Input: part model. Units: mm. Frame: model coordinates. Face numbers are marked on the shaded views. A direction names the side the tool comes from. Round coordinates to 2 decimals unless told otherwise and drop trailing zeros. Write each loop counter-clockwise with the first axis right and the second up, starting at its lowest first coordinate (ties: lowest second). Pieces come first, ordered by that corner, then holes. Notation, with made-up numbers: (11, -22) -> (28, -22) arc R24 cw to (28, 4) -> close; hole circle Ø5 at (65, -19). An arc over 180 degrees is marked (long way). Use CSV: the item, a comma, the result in double quotes.
```python
from build123d import *

# Parameters (mm, degrees)
BOSS_EXTRUDE1_DEPTH = 38.1
SKETCH2_W           = 28.575
SKETCH2_H           = 22.225
CUT_EXTRUDE1_DEPTH  = 39.1
SKETCH3_R           = 1.5875
CUT_EXTRUDE2_DEPTH  = 37.5125
SKETCH4_R           = 1.8415
CUT_EXTRUDE3_DEPTH  = 37.5125
CIRPATTERN1_COUNT   = 8
FILLET1_R           = 2.54
FILLET2_R           = 2.54


with BuildPart() as part:
    # Sketch1 → Boss-Extrude1 (new body)
    with BuildSketch(Plane.XY):
        Polygon((0, 0), (0, 31.75), (33.3375, 31.75), (33.3375, 36.5125), (-4.7625, 36.5125), (-4.7625, 0), align=None)
    extrude(amount=BOSS_EXTRUDE1_DEPTH)

    # Sketch2 → Cut-Extrude1 (cut, through all)
    with BuildSketch(Plane.ZY.offset(4.7625)):
        with Locations((19.05, 14.2875)):
            Rectangle(SKETCH2_W, SKETCH2_H)
    extrude(amount=-CUT_EXTRUDE1_DEPTH, mode=Mode.SUBTRACT)

    # Sketch3 → Cut-Extrude2 (cut, through all)
    with BuildSketch(Plane(origin=(0, 36.5125, 0), x_dir=(1, 0, 0), z_dir=(0, 1, 0))):
        with Locations((17.4625, -19.05)):
            Circle(SKETCH3_R)
    extrude(amount=-CUT_EXTRUDE2_DEPTH, mode=Mode.SUBTRACT)

    # Sketch4 → Cut-Extrude3 (cut, through all)
    with BuildSketch(Plane(origin=(0, 36.5125, 0), x_dir=(1, 0, 0), z_dir=(0, 1, 0))):
        with Locations((27.2415, -19.05)):
            Circle(SKETCH4_R)
    cut_extrude3 = extrude(amount=-CUT_EXTRUDE3_DEPTH, mode=Mode.SUBTRACT)

    # CirPattern1: Cut-Extrude3 ×8 about axis
    cirpattern1_axis = Axis((17.4625, 0, 19.05), (0, 1, 0))
    for i in range(1, CIRPATTERN1_COUNT):
        add(cut_extrude3.rotate(cirpattern1_axis, i * 360 / CIRPATTERN1_COUNT), mode=Mode.SUBTRACT)

    # Fillet1
    fillet1_edges = [part.edges().sort_by_distance(p)[0] for p in [
        (0, 31.75, 19.05),
    ]]
    fillet(fillet1_edges, radius=FILLET1_R)

    # Fillet2
    fillet2_edges = [part.edges().sort_by_distance(p)[0] for p in [
        (33.3375, 34.13125, 38.1),
        (-2.38125, 0, 38.1),
        (33.3375, 34.13125, 0),
        (-2.38125, 0, 0),
    ]]
    fillet(fillet2_edges, radius=FILLET2_R)


solid = part.part
```
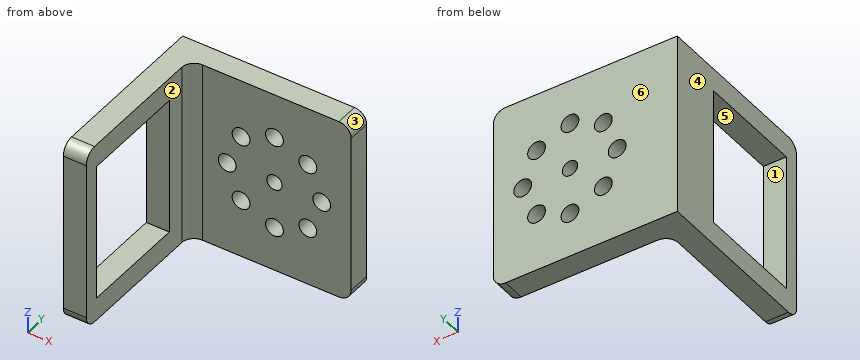
Item 1: Section query D-D on x = 8. Return the cut outline in (y, z).
Worked answers:
outline,"(31.75, 0) -> (36.51, 0) -> (36.51, 17.24) -> (31.75, 17.24) -> close; (31.75, 20.86) -> (36.51, 20.86) -> (36.51, 38.1) -> (31.75, 38.1) -> close"
Item 2: First-contact query: pin 1 Ø6 at (x, z) = (15, 11) entering from -Y; pin 2 Ø3.5 at (x, z) = (27.24, 19.05) entering from -Y; pin 3 Ø4 at (x, z) = (10.55, 25.96) entering from +Y; pin 4 Ø10 at (y, z) = (4, 24) entering from +X. Flat tips, straight axial feed; report the tip coordinate or a pass-through.
Worked answers:
pin 1,"stops at y = 31.75"
pin 2,"passes through"
pin 3,"stops at y = 36.51"
pin 4,"stops at x = 0"
Item 3: Line query: line 1 (Y direction, x = 7, z = 16); line 2 (Y direction, x = -3, z = 15.5) (1 decimal); line 3 (X direction, y = 2, z = 34). Output: solid intervals per line, ascending.
Worked answers:
line 1,"y = 31.75 to 36.51"
line 2,"y = 0 to 3.2, 25.4 to 36.5"
line 3,"x = -4.76 to 0"
Item 4: Section query C-C on z = 19.05. Give the number of separate pieces and of enclosed holes in the cut face, plus the area to 3 significant figures.
Worked answers:
separate pieces,"5"
enclosed holes,"0"
area,"178 mm²"
Item 5: Pull-direction query (Y, two-part tool) for the marked faces 4, 5 and 6; classes: +Y half, -Y half, draft (parallel to the pull), parting line (faces both ways), or undercut.
Worked answers:
face 4,"draft"
face 5,"undercut"
face 6,"+Y half"
Item 6: Section query B-B on y = 24. Return the cut outline in (x, z).
Worked answers:
outline,"(-4.76, 0) -> (0, 0) -> (0, 4.76) -> (-4.76, 4.76) -> close; (-4.76, 33.34) -> (0, 33.34) -> (0, 38.1) -> (-4.76, 38.1) -> close"
Item 7: Set-up query: the marked faces 1, 2 and 3. Return all of +Z, -Z, +X, -X, +Y, -Y with unobstructed straight access to the full face (end or side cutting, diameter ignored); none if empty.
Worked answers:
face 1,"+X, -X"
face 2,"+Z, -Z, +X, -Y"
face 3,"+Z, +X, +Y, -Y"
